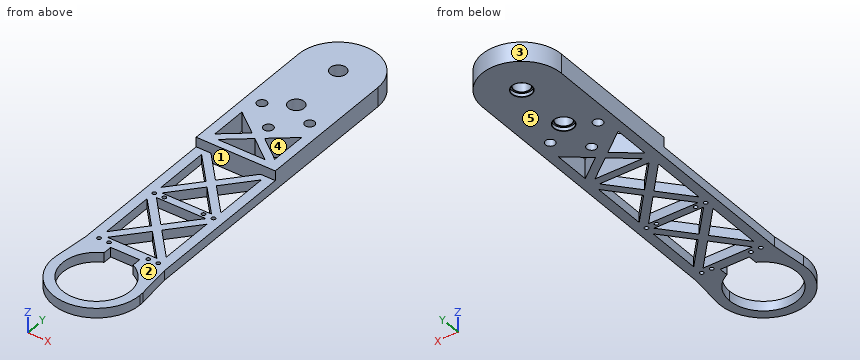
```python
from build123d import *

# Parameters (mm, degrees)
SKETCH_1_R               = 20.5
SKETCH_1_R_2             = 6.5
SKETCH_1_R_3             = 1.5
EXTRUDE_1_DEPTH          = 10
SKETCH_2_R               = 4.1
CUT_EXTRUDE_1_DEPTH      = 10
SKETCH_4_W               = 41
SKETCH_4_H               = 120.125
CUT_EXTRUDE_3_DEPTH      = 5
CUT_EXTRUDE_4_DEPTH      = 195.839677684
CUT_EXTRUDE_4_DEPTH_BACK = 10
CUT_EXTRUDE_5_DEPTH      = 195.839677684
CUT_EXTRUDE_5_DEPTH_BACK = 10
SKETCH_5_W               = 41
SKETCH_5_H               = 41
CUT_EXTRUDE_6_DEPTH      = 10
EXTRUDE_START            = -5
EXTRUDE_2_DEPTH          = 5
SKETCH_7_R               = 1
CUT_EXTRUDE_7_DEPTH      = 195.867903976
SKETCH_8_R               = 2.5
CUT_EXTRUDE_8_DEPTH      = 10
CUT_EXTRUDE_START        = -10
SKETCH_9_R               = 5
CUT_EXTRUDE_9_DEPTH      = 1.8
FILLET_1_R               = 0.2


with BuildPart() as part:
    # 스케치1 → 보스-돌출1 (new body)
    # profile 1 of 3: a face of its own
    with BuildSketch(Plane.XY):
        with BuildLine():
            Line((-20.5, 173), (-20.5, 0))
            ThreePointArc((-20.5, 0), (0, 20.5), (20.5, 0))
            Line((20.5, 0), (20.5, 173))
            ThreePointArc((20.5, 173), (0, 152.5), (-20.5, 173))
        make_face()
    # profile 2 of 3: a face of its own
    with BuildSketch(Plane.XY):
        with Locations((0, 173)):
            Circle(SKETCH_1_R)
    # profile 3 of 3: a face of its own
    with BuildSketch(Plane.XY):
        Circle(SKETCH_1_R)
        with Locations((0, -7)):
            Circle(SKETCH_1_R_2, mode=Mode.SUBTRACT)
        with Locations((-7.75, -13.423393759)):
            Circle(SKETCH_1_R_3, mode=Mode.SUBTRACT)
        with Locations((7.75, -13.423393759)):
            Circle(SKETCH_1_R_3, mode=Mode.SUBTRACT)
        with Locations((15.5, 0)):
            Circle(SKETCH_1_R_3, mode=Mode.SUBTRACT)
        with Locations((7.75, 13.423393759)):
            Circle(SKETCH_1_R_3, mode=Mode.SUBTRACT)
        with Locations((-7.75, 13.423393759)):
            Circle(SKETCH_1_R_3, mode=Mode.SUBTRACT)
        with Locations((-15.5, 0)):
            Circle(SKETCH_1_R_3, mode=Mode.SUBTRACT)
    extrude(amount=-EXTRUDE_1_DEPTH)

    # 스케치2 → 컷-돌출1 (cut)
    with BuildSketch(Plane.XY):
        with Locations((0, 173)):
            Circle(SKETCH_2_R)
        with Locations((0, 143)):
            Circle(SKETCH_2_R)
    extrude(amount=-CUT_EXTRUDE_1_DEPTH, mode=Mode.SUBTRACT)

    # 스케치4 → 컷-돌출3 (cut)
    with BuildSketch(Plane.XY):
        with Locations((0, 39.5625)):
            Rectangle(SKETCH_4_W, SKETCH_4_H)
    extrude(amount=-CUT_EXTRUDE_3_DEPTH, mode=Mode.SUBTRACT)

    # 스케치3 → 컷-돌출4 (cut, two sides: drawn at the far end of the back side and taken through both)
    with BuildSketch(Plane.XY.offset(-CUT_EXTRUDE_4_DEPTH_BACK)):
        Polygon((15.5, 125.455788946), (3.235714571, 115.8125), (15.5, 106.169211054), align=None)
        Polygon((12.264285429, 103.625), (0, 113.268288946), (-12.264285429, 103.625), align=None)
        Polygon((-3.235714571, 115.8125), (-15.5, 125.455788946), (-15.5, 106.169211054), align=None)
    extrude(amount=CUT_EXTRUDE_4_DEPTH + CUT_EXTRUDE_4_DEPTH_BACK, mode=Mode.SUBTRACT)

    # 스케치3<4> → 컷-돌출5 (cut, two sides: drawn at the far end of the back side and taken through both)
    with BuildSketch(Plane.XY.offset(-CUT_EXTRUDE_5_DEPTH_BACK)):
        Polygon((12.830480138, 99.625), (-12.830480138, 99.625), (0, 85.112071418), align=None)
        Polygon((15.5, 67.579571418), (15.5, 96.605428582), (2.669519862, 82.0925), align=None)
        Polygon((12.830480138, 64.56), (0, 79.072928582), (-12.830480138, 64.56), align=None)
        Polygon((-2.669519862, 82.0925), (-15.5, 96.605428582), (-15.5, 67.579571418), align=None)
        Polygon((12.830313114, 60.56), (-12.830313114, 60.56), (0, 46.049329749), align=None)
        Polygon((-2.669686886, 43.03), (-15.5, 57.540670251), (-15.5, 28.519329749), align=None)
        Polygon((12.830313114, 25.5), (0, 40.010670251), (-12.830313114, 25.5), align=None)
        Polygon((15.5, 28.519329749), (15.5, 57.540670251), (2.669686886, 43.03), align=None)
    extrude(amount=CUT_EXTRUDE_5_DEPTH + CUT_EXTRUDE_5_DEPTH_BACK, mode=Mode.SUBTRACT)

    # 스케치5 → 컷-돌출6 (cut)
    with BuildSketch(Plane.XY):
        Rectangle(SKETCH_5_W, SKETCH_5_H)
    extrude(amount=-CUT_EXTRUDE_6_DEPTH, mode=Mode.SUBTRACT)

    # 스케치6 → 보스-돌출2 (add)
    with BuildSketch(Plane.XY.offset(EXTRUDE_START)):
        with BuildLine():
            ThreePointArc((-22.380643152, 2.314478799), (-18.253119335, 13.155745306), (-9.273618495, 20.5))
            Line((-9.273618495, 20.5), (-20.5, 20.5))
            Line((-20.5, 20.5), (-22.380643152, 2.314478799))
        make_face()
        with BuildLine():
            Line((-7.5, 15.811388301), (-7.5, 20.5))
            Line((-7.5, 20.5), (-9.273618495, 20.5))
            ThreePointArc((-9.273618495, 20.5), (-18.253119335, 13.155745306), (-22.380643152, 2.314478799))
            ThreePointArc((-22.380643152, 2.314478799), (-1.158777176, -22.470140975), (22.5, 0))
            ThreePointArc((22.5, 0), (22.470140975, 1.158777176), (22.380643152, 2.314478799))
            ThreePointArc((22.380643152, 2.314478799), (18.253119335, 13.155745306), (9.273618495, 20.5))
            Line((9.273618495, 20.5), (7.5, 20.5))
            Line((7.5, 20.5), (7.5, 15.811388301))
            ThreePointArc((7.5, 15.811388301), (14.790199458, 9.354143467), (17.5, 0))
            ThreePointArc((17.5, 0), (-9.354143467, -14.790199458), (-7.5, 15.811388301))
        make_face()
        with BuildLine():
            Line((20.5, 20.5), (9.273618495, 20.5))
            ThreePointArc((9.273618495, 20.5), (18.253119335, 13.155745306), (22.380643152, 2.314478799))
            Line((22.380643152, 2.314478799), (20.5, 20.5))
        make_face()
    extrude(amount=-EXTRUDE_2_DEPTH)

    # 스케치7 → 컷-돌출7 (cut, through all)
    with BuildSketch(Plane.XY.offset(-5)):
        with Locations((-15.33, 23)):
            Circle(SKETCH_7_R)
        with Locations((-10.16, 23)):
            Circle(SKETCH_7_R)
        with Locations((10.16, 23)):
            Circle(SKETCH_7_R)
        with Locations((15.33, 23)):
            Circle(SKETCH_7_R)
        with Locations((-15.33, 62.56)):
            Circle(SKETCH_7_R)
        with Locations((-10.16, 62.56)):
            Circle(SKETCH_7_R)
        with Locations((10.16, 62.56)):
            Circle(SKETCH_7_R)
        with Locations((15.33, 62.56)):
            Circle(SKETCH_7_R)
    extrude(amount=-CUT_EXTRUDE_7_DEPTH, mode=Mode.SUBTRACT)

    # 스케치8 → 컷-돌출8 (cut)
    with BuildSketch(Plane.XY):
        with Locations((-12.37, 135.5)):
            Circle(SKETCH_8_R)
        with Locations((0, 123)):
            Circle(SKETCH_8_R)
        with Locations((12.37, 135.5)):
            Circle(SKETCH_8_R)
    extrude(amount=-CUT_EXTRUDE_8_DEPTH, mode=Mode.SUBTRACT)

    # 스케치9 → 컷-돌출9 (cut)
    with BuildSketch(Plane.XY.offset(CUT_EXTRUDE_START)):
        with Locations((0, 173)):
            Circle(SKETCH_9_R)
        with Locations((0, 143)):
            Circle(SKETCH_9_R)
    extrude(amount=CUT_EXTRUDE_9_DEPTH, mode=Mode.SUBTRACT)

    # 필렛1
    fillet_1_edges = [part.edges().sort_by_distance(p)[0] for p in [
        (-4.1, 173, -8.2),
        (-5, 173, -10),
        (-4.1, 143, -8.2),
        (-5, 143, -10),
    ]]
    fillet(fillet_1_edges, radius=FILLET_1_R)


solid = part.part
```
The model under review builds one solid part; all positions refer to its coordinate system, in mm. Face numbers are marked on the shaded views. A direction names the side the tool comes from. Round coordinates to 2 decimals unless told otherwise and drop trailing zeros. Loops run counter-clockwise (first coordinate to the right, second up) from the corner with the lowest first, then second, coordinate; pieces in that order, holes last. Notation, with made-up numbers: (58, 56.5) - (84, 56.5) arc R4 ccw to (84, 62.5) - close; hole circle Ø8 at (71.5, -5). An arc over 180 degrees is marked (long way). Use a Markdown table: item, result. Add a question column.
Q1. The part is to be moulded in two halves that separate along X. For the marked faces 1, 2 and 3, say which applies: pulls with the +X half, pulls with the -X half, needs draft (parallel to the pull), parting line crosses it, or undercut.
Q2. Machinability: for the marked faces 4 and 5, which of the approach directions +Z, -Z, +X, -X, +Y, -Y give a long, thin tool a straight path to every point of the face, cutting with its end or side? Answer none if there is none.
Q3. Add section B-B (y = 9.5). State the section outline as (x, z) points.
Q4. For probe 1 along Y at (x, z) = (-11.5, -2.25) (3 decimals); probe 2 along X at (y, z) = (43.5, -6.5); probe 3 along Z at (x, y) = (17.5, 86), list the stretches that pass through material, from the lowest coordinate up.
Q5. Insertion check: pin 1 Ø2.5 at (x, y) = (15.33, 62.56) entering from -Z; pin 2 Ø5 at (x, z) = (2, -2.5) entering from +Y; pin 3 Ø13.5 at (x, y) = (-3.5, 24.5) entering from +Z; pin 4 Ø6 at (x, y) = (0, 143) entering from +Z. Each pin has a flat end and moves straight along its axis. Give the tip position at first contact, or say it passes through.
Q6. Add section A-A (z = -1.5). State how many separate pieces and enclosed holes the cut face has, plus the area to 3 significant figures.
Q7. Add section D-D (y = 180). State the section outline as (x, z) points, plus the area to 3 significant figures.
Q8. Add section C-C (y = 123). State the section outline as (x, z) points.
Worked answers:
| question | item | result |
|---|---|---|
| 1 | face 1 | undercut |
| 1 | face 2 | needs draft |
| 1 | face 3 | parting line crosses it |
| 2 | face 4 | +Z, -Z |
| 2 | face 5 | -Z, +X, -X, +Y, -Y |
| 3 | outline | (-21.64, -10) - (-14.7, -10) - (-14.7, -5) - (-21.64, -5) - close; (14.7, -10) - (21.64, -10) - (21.64, -5) - (14.7, -5) - close |
| 4 | probe 1 | 99.625 to 103.625, 104.226 to 109.314, 122.311 to 133.156, 137.844 to 189.971 |
| 4 | probe 2 | -20.5 to -15.5, -3.09 to 3.09, 15.5 to 20.5 |
| 4 | probe 3 | -10 to -5 |
| 5 | pin 1 | z = -10 |
| 5 | pin 2 | y = 193.5 |
| 5 | pin 3 | z = -5 |
| 5 | pin 4 | through |
| 6 | separate pieces | 1 |
| 6 | enclosed holes | 8 |
| 6 | area | 3,150 mm² |
| 7 | outline | (-19.27, -10) - (19.27, -10) - (19.27, 0) - (-19.27, 0) - close |
| 7 | area | 385 mm² |
| 8 | outline | (-20.5, -10) - (-15.5, -10) - (-15.5, 0) - (-20.5, 0) - close; (-12.38, -10) - (-2.5, -10) - (-2.5, 0) - (-12.38, 0) - close; (2.5, -10) - (12.38, -10) - (12.38, 0) - (2.5, 0) - close; (15.5, -10) - (20.5, -10) - (20.5, 0) - (15.5, 0) - close |
